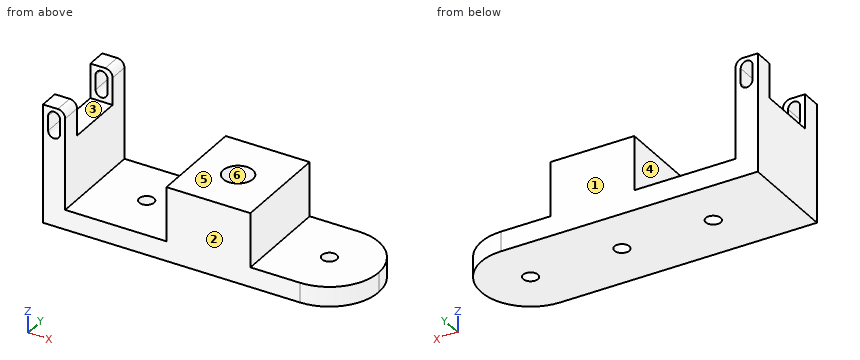
```python
from build123d import *

# Parameters (mm, degrees)
SKETCH_1_W          = 57
SKETCH_1_H          = 20
SKETCH_1_R          = 1.5
EXTRUDE_1_DEPTH     = 4
FILLET_1_R          = 10
SKETCH_4_W          = 17
SKETCH_4_H          = 20
EXTRUDE_3_DEPTH     = 11
SKETCH_5_R          = 3
CUT_EXTRUDE_1_DEPTH = 9
SKETCH_6_R          = 1.5
CUT_EXTRUDE_2_DEPTH = 6
SKETCH_7_W          = 4
SKETCH_7_H          = 20
EXTRUDE_4_DEPTH     = 5
SKETCH_8_W          = 4.5
SKETCH_8_H          = 20
EXTRUDE_5_DEPTH     = 13
SKETCH_9_W          = 4.5
SKETCH_9_H          = 4
EXTRUDE_6_DEPTH     = 7
CUT_EXTRUDE_START   = -20
CUT_EXTRUDE_3_DEPTH = 20
FILLET_2_R          = 1.5


with BuildPart() as part:
    # 草图1 → 凸台-拉伸1 (new body)
    with BuildSketch(Plane.XY):
        Rectangle(SKETCH_1_W, SKETCH_1_H)
        with Locations((-18.5, 0)):
            Circle(SKETCH_1_R, mode=Mode.SUBTRACT)
        with Locations((18.5, 0)):
            Circle(SKETCH_1_R, mode=Mode.SUBTRACT)
    extrude(amount=EXTRUDE_1_DEPTH)

    # 圆角1
    fillet_1_edges = [part.edges().sort_by_distance(p)[0] for p in [
        (28.5, -10, 2),
        (28.5, 10, 2),
    ]]
    fillet(fillet_1_edges, radius=FILLET_1_R - 0.0001)  # a hair under: the kernel refuses the full size

    # 草图4 → 凸台-拉伸3 (add)
    with BuildSketch(Plane.XY.offset(4)):
        Rectangle(SKETCH_4_W, SKETCH_4_H)
    extrude(amount=EXTRUDE_3_DEPTH)

    # 草图5 → 切除-拉伸1 (cut)
    with BuildSketch(Plane.XY.offset(15)):
        Circle(SKETCH_5_R)
    extrude(amount=-CUT_EXTRUDE_1_DEPTH, mode=Mode.SUBTRACT)

    # 草图6 → 切除-拉伸2 (cut)
    with BuildSketch(Plane.XY.offset(6)):
        Circle(SKETCH_6_R)
    extrude(amount=-CUT_EXTRUDE_2_DEPTH, mode=Mode.SUBTRACT)

    # 草图7 → 凸台-拉伸4 (add)
    with BuildSketch(Plane.ZY.offset(28.5)):
        with Locations((2, 0)):
            Rectangle(SKETCH_7_W, SKETCH_7_H)
    extrude(amount=EXTRUDE_4_DEPTH)

    # 草图8 → 凸台-拉伸5 (add)
    with BuildSketch(Plane.XY.offset(4)):
        with Locations((-31.25, 0)):
            Rectangle(SKETCH_8_W, SKETCH_8_H)
    extrude(amount=EXTRUDE_5_DEPTH)

    # 草图9 → 凸台-拉伸6 (add)
    with BuildSketch(Plane.XY.offset(17)):
        with Locations((-31.25, 8)):
            Rectangle(SKETCH_9_W, SKETCH_9_H)
        with Locations((-31.25, -8)):
            Rectangle(SKETCH_9_W, SKETCH_9_H)
    extrude(amount=EXTRUDE_6_DEPTH)

    # 草图10 → 切除-拉伸3 (cut)
    with BuildSketch(Plane(origin=(0, 10, 0), x_dir=(1, 0, 0), z_dir=(0, 1, 0)).offset(CUT_EXTRUDE_START)):
        with BuildLine():
            Line((-32.45, -22), (-32.45, -19))
            ThreePointArc((-32.45, -19), (-31.25, -17.8), (-30.05, -19))
            Line((-30.05, -19), (-30.05, -22))
            ThreePointArc((-30.05, -22), (-31.25, -23.2), (-32.45, -22))
        make_face()
    extrude(amount=CUT_EXTRUDE_3_DEPTH, mode=Mode.SUBTRACT)

    # 圆角2
    fillet_2_edges = [part.edges().sort_by_distance(p)[0] for p in [
        (-29, 8, 24),
        (-29, -8, 24),
    ]]
    fillet(fillet_2_edges, radius=FILLET_2_R)


solid = part.part
```
Could you check a few things on this model? Use its own coordinates, in mm. Face numbers are marked on the shaded views. A direction names the side the tool comes from. Round coordinates to 2 decimals unless told otherwise and drop trailing zeros. Loops run counter-clockwise (first coordinate to the right, second up) from the corner with the lowest first, then second, coordinate; pieces in that order, holes last. Notation, with made-up numbers: M 7,19 L 20,19 A14 ccw 20,26 Z; hole C 23.5,65 d11. An arc over 180 degrees is marked long. Write item = value, one per line.
1. I want a section at A-A, the plane z = 8.75. Write out the boundary of the cut face in (x, y).
Results below:
outline = M -33.5,-10 L -29,-10 L -29,10 L -33.5,10 Z; M -8.5,-10 L 8.5,-10 L 8.5,10 L -8.5,10 Z; hole C 0,0 d6
2. I want a section at D-D, the plane y = 0.75. Write out the boundary of the cut face in (x, z).
Results below:
outline = M -33.5,0 L -19.8,0 L -19.8,4 L -29,4 L -29,17 L -33.5,17 Z; M -17.2,0 L -1.3,0 L -1.3,6 L -2.9,6 L -2.9,15 L -8.5,15 L -8.5,4 L -17.2,4 Z; M 1.3,0 L 17.2,0 L 17.2,4 L 8.5,4 L 8.5,15 L 2.9,15 L 2.9,6 L 1.3,6 Z; M 19.8,0 L 28.47,0 L 28.47,4 L 19.8,4 Z
3. I want a section at B-B, the plane x = -18.5. Write out the boundary of the cut face in (y, z), and give its area (3 significant figures).
Results below:
outline = M -10,0 L -1.5,0 L -1.5,4 L -10,4 Z; M 1.5,0 L 10,0 L 10,4 L 1.5,4 Z
area = 68.0 mm²
4. Will these pins go through, and if not, where does the flat tip stop? P1, Ø0.9, axis at y = -8.5, z = 20, coming from the +X side; P2, Ø5.5, axis at y = 1, z = 11.5, coming from the +X side; P3, Ø6, axis at x = 21.5, y = 5, coming from the +Z side.
Results below:
P1 = -29
P2 = 8.5
P3 = 4
5. Which directions (+Z, -Z, +X, -X, +Y, -Y) give clear straight access to the entire face, cutting with the end or side of a thin tool? Please do the marked faces 4, 5 and 6.
Results below:
face_4 = +Z, +Y, -Y
face_5 = +Z, +X, +Y, -Y
face_6 = +Z
6. I want a section at C-C, the plane x = -31.25. Write out the boundary of the cut face in (y, z), and give its area (3 significant figures).
Results below:
outline = M -10,0 L 10,0 L 10,17.8 L 6,17.8 L 6,17 L -6,17 L -6,17.8 L -10,17.8 Z; M -10,23.2 L -6,23.2 L -6,24 L -10,24 Z; M 6,23.2 L 10,23.2 L 10,24 L 6,24 Z
area = 353 mm²
7. I need wall thicknesses on probe 1 along Y at (x, z) = (-18.5, 1.25); probe 2 along X at (y, z) = (-6, 14); probe 3 along Z at (x, y) = (22.5, -5.75). Which ranges of each line are inside material? Lowest first, please.
Results below:
probe_1 = -10 to -1.5, 1.5 to 10
probe_2 = -33.5 to -29, -8.5 to 8.5
probe_3 = 0 to 4
8. Thinking about a two-plate mould opening in Y: for the marked faces 1, 2 and 3, which applies, +Y half, -Y half, draft (parallel to the pull), parting line (faces both ways), or undercut?
Results below:
face_1 = +Y half
face_2 = -Y half
face_3 = undercut
